Work out the finished part from the listing and answer in its coordinate system (mm). Round coordinates to 2 decimals unless told otherwise and drop trailing zeros. Write each loop counter-clockwise with the first axis right and the second up, starting at its lowest first coordinate (ties: lowest second). Pieces come first, ordered by that corner, then holes. Notation, with made-up numbers: (58.5, 17.5) - (68.5, 17.5) arc R27 cw to (68.5, 47.5) - close; hole circle Ø5 at (36, -10). An arc over 180 degrees is marked (long way). Write item = value, one per line. Start each with the question number.
from build123d import *

# Parameters (mm, degrees)
F0_W     = 60
F0_H     = 30
F1_DEPTH = 15
F2_R     = 10
F3_DEPTH = 30
F3_TAPER = 18


with BuildPart() as f1:
    # F0 (on Top) → F1 (new body)
    with BuildSketch(Plane.XY):
        with Locations((30, 15)):
            Rectangle(F0_W, F0_H)
    extrude(amount=F1_DEPTH)

    # F2 (on face) → F3 (join)
    with BuildSketch(Plane.XY.offset(15)):
        with Locations((36.5466400981, 15)):
            Circle(F2_R)
    extrude(amount=F3_DEPTH, taper=F3_TAPER)


solid = f1.part
1. Each of these flat-tipped pins is pushed along its axis until it touches: pin 1 (8 mm diameter, centred on x = 33, y = 18.5, fed in from -Z); pin 2 (1 mm diameter, centred on x = 20.5, y = 22.5, fed in from +Z); pin 3 (4 mm diameter, centred on x = 29, z = 18, fed in from +Y); pin 4 (1 mm diameter, centred on y = 9.5, z = 17, fed in from +X). Where does it stop, or does it pass through?
2. Find section D-D on z = 35. Give the vertices of the cut face in (x, y), plus the area to 3 significant figures.
3. Find section B-B on x = 11.5. Give the vertices of the cut face in (y, z), plus the area to 3 significant figures.
4. Find section A-A on y = 26. Give the vertices of the cut face in (x, z), plus the area to 3 significant figures.
5. Find section C-C on z = 24. Give the vertices of the cut face in (x, y), plus the area to 3 significant figures.
6. Consider line 1 (Z direction, x = 56, y = 16.5); line 2 (X direction, y = 17.75, z = 29.5); line 3 (X direction, y = 12, z = 26.5). Determine where each line is inside the solid, lowest interval first.
Answer key:
q1.pin_1 = 0
q1.pin_2 = 15
q1.pin_3 = 22.32
q1.pin_4 = 44.5
q2.outline = circle Ø7 at (36.55, 15)
q2.area = 38.5 mm²
q3.outline = (0, 0) - (30, 0) - (30, 15) - (0, 15) - close
q3.area = 450 mm²
q4.outline = (0, 0) - (60, 0) - (60, 15) - (0, 15) - close
q4.area = 900 mm²
q5.outline = circle Ø14.15 at (36.55, 15)
q5.area = 157 mm²
q6.line_1 = 0 to 15
q6.line_2 = 32.03 to 41.06
q6.line_3 = 31.05 to 42.04
